The drawing under review shows one solid part. Ordinate dimensions are in mm from its lowest x, y, z. A direction names the side the tool comes from. Round coordinates to 2 decimals unless told otherwise and drop trailing zeros. Order: outer loops, then holes, each group sorted by start corner. A loop starts at its lowest first (then second) coordinate and runs counter-clockwise, first axis right, second up.
1) Clearance check with flat-ended pins moving along their axes: P1, Ø2, axis at x = 3.5, y = 35, coming from the +Z side (3 decimals); P2, Ø1, axis at y = 20, z = 2.5, coming from the -X side. State where each tip first meets the part, or that it passes through.
2) To check wall thickness, follow L1, parallel to Z at x = 3, y = 13.5; L2, parallel to Y at x = 6, z = 1. State the ranges of each line that lie inside material, in increasing order.
3) Consider section C-C (y = 4). Give the boundary of the cut face in (x, z) (3 decimals).
4) Consider section A-A (x = 2.5). Give the boundary of the cut face in (y, z).
5) Machinability: for the marked faces 1, 2 and 3, which of the approach directions +Z, -Z, +X, -X, +Y, -Y give a long, thin tool a straight path to every point of the face, cutting with its end or side? Answer none if there is none.
6) Consider section B-B (z = 2.25). Give the boundary of the cut face in (x, y).
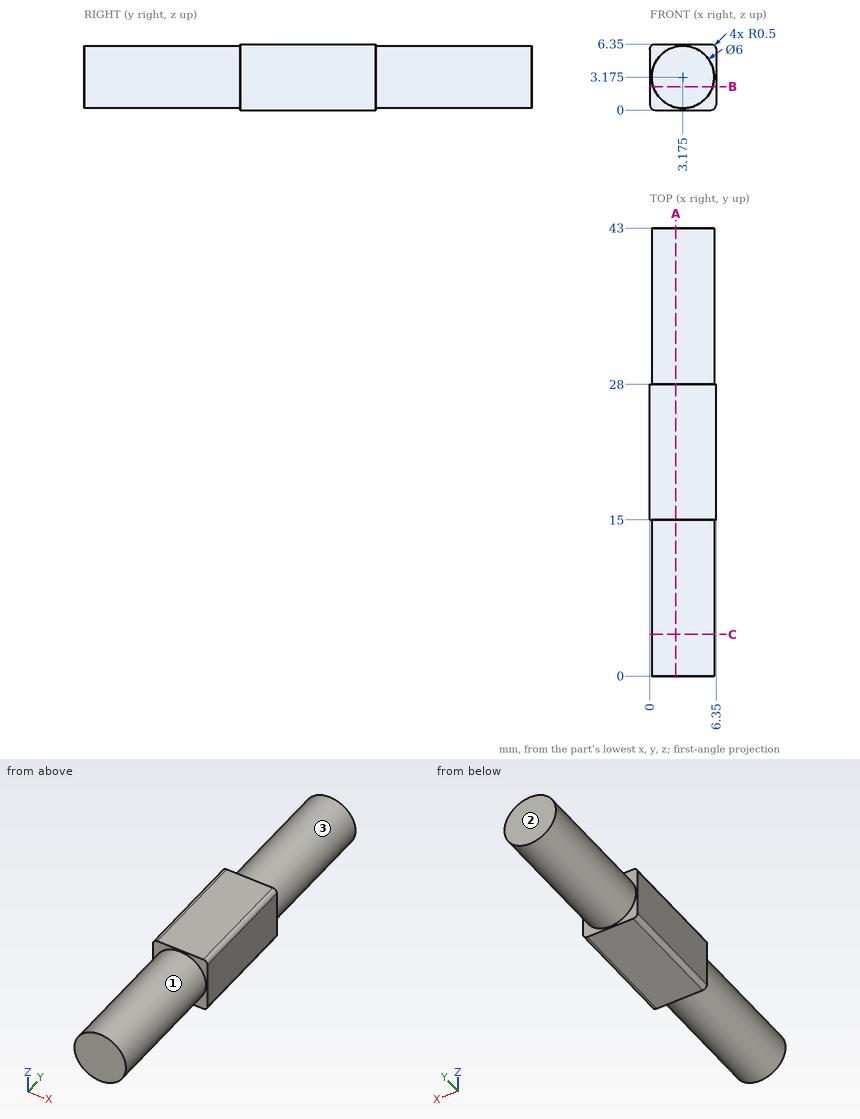
Answer below:
1. P1: stops at z = 6.175
1. P2: stops at x = 0
2. L1: z = 0.18 to 6.17
2. L2: y = 15 to 28
3. outline: circle Ø6 at (3.175, 3.175)
4. outline: (0, 0.25) - (15, 0.25) - (15, 0) - (28, 0) - (28, 0.25) - (43, 0.25) - (43, 6.1) - (28, 6.1) - (28, 6.35) - (15, 6.35) - (15, 6.1) - (0, 6.1) - close
5. face 1: -Y
5. face 2: +Z, -Z, +X, -X, +Y
5. face 3: +Y
6. outline: (0, 15) - (0.32, 15) - (0.32, 0) - (6.03, 0) - (6.03, 15) - (6.35, 15) - (6.35, 28) - (6.03, 28) - (6.03, 43) - (0.32, 43) - (0.32, 28) - (0, 28) - close
